Read the model definition and answer for the solid it produces. Units are mm, in the model's axes. A direction names the side the tool comes from. Coordinates: 2 decimals unless noted, no trailing zeros. Write each loop counter-clockwise with the first axis right and the second up, starting at its lowest first coordinate (ties: lowest second). Pieces come first, ordered by that corner, then holes. Notation, with made-up numbers: M 55,31.5 L 81,31.5 A22 ccw 81,41.5 Z; hole C 8,-35 d4. An arc over 180 degrees is marked long. Write item = value, one per line.
from build123d import *

# Parameters (mm, degrees)
F0_R     = 4.5
F1_DEPTH = 8
F2_W     = 22
F2_H     = 60
F2_R     = 2.5
F3_DEPTH = 6
F4_SIZE  = 1


with BuildPart() as f1:
    # F0 (on Right) → F1 (new body, symmetric)
    with BuildSketch(Plane.YZ):
        with BuildLine():
            Line((-30, 10), (-10.925823, -10.27747))
            ThreePointArc((-10.925823, -10.27747), (0, -15), (10.925823, -10.27747))
            Line((10.925823, -10.27747), (30, 10))
            Line((30, 10), (30, 20))
            Line((30, 20), (0, 20))
            Line((0, 20), (-30, 20))
            Line((-30, 20), (-30, 10))
        make_face()
        Circle(F0_R, mode=Mode.SUBTRACT)
    extrude(amount=F1_DEPTH, both=True)

    # F2 (on face) → F3 (join)
    with BuildSketch(Plane.XY.offset(20)):
        Polygon((8, 30), (0, 30), (-8, 30), (-8, -30), (8, -30), align=None)
        with Locations((19, 0)):
            Rectangle(F2_W, F2_H)
        with Locations((20, -20)):
            Circle(F2_R, mode=Mode.SUBTRACT)
        with Locations((20, 20)):
            Circle(F2_R, mode=Mode.SUBTRACT)
        with Locations((-19, 0)):
            Rectangle(F2_W, F2_H)
        with Locations((-20, -20)):
            Circle(F2_R, mode=Mode.SUBTRACT)
        with Locations((-20, 20)):
            Circle(F2_R, mode=Mode.SUBTRACT)
    extrude(amount=F3_DEPTH)

    # F4
    f4_edges = [f1.edges().sort_by_distance(p)[0] for p in [
        (0, 30, 26),
        (-30, 0, 26),
        (0, -30, 26),
        (30, 0, 26),
        (17.5, 20, 26),
        (17.5, -20, 26),
        (-22.5, 20, 26),
        (-22.5, -20, 26),
    ]]
    chamfer(f4_edges, length=F4_SIZE)


solid = f1.part
Item 1: Consider line 1 along Y through (x, z) = (20, 23.95); line 2 along Z through (x, y) = (21.5, -27); line 3 along Z through (x, y) = (-6, -1). Determine where each line is inside the solid, lowest interval first. Write a range as from..to.
Worked answers:
line_1 = -30..-22.5, -17.5..17.5, 22.5..30
line_2 = 20..26
line_3 = -14.97..-4.39, 4.39..26
Item 2: Flat-ended cylindrical pins translate along their axes: pin 1 (2 mm diameter, centred on x = 6.5, y = 20, fed in from -Z); pin 2 (6.5 mm diameter, centred on x = 21, y = -12, fed in from -Z); pin 3 (8 mm diameter, centred on y = 10, z = -9.5, fed in from +X); pin 4 (8 mm diameter, centred on x = -20, y = -20, fed in from +Z). Find the tip coordinate at first contact, or state that the pin passes through.
Worked answers:
pin_1 = -1.69
pin_2 = 20
pin_3 = 8
pin_4 = 26
Item 3: For a pull along X with two mould halves and no side action, classify faces 4 (the face through (-8, 0, 7)), 5 (the face through (-21.84, 21.69, 22.46)), 6 (the face through (0, -30, 19)), 7 (the face through (30, 0, 22)) as released by +X, released by -X, zero draft, split by the parting line, or undercut.
Worked answers:
face_4 = released by -X
face_5 = undercut
face_6 = zero draft
face_7 = released by +X
Item 4: Which of the six approach directions +Z, -Z, +X, -X, +Y, -Y give full straight-line access (tool end or side, diameter ignored) to faces 1 (the face through (-19, 0, 20)), 2 (the face through (8, 0, 7)), 3 (the face through (-30, 0, 22))?
Worked answers:
face_1 = -Z, -X, +Y, -Y
face_2 = -Z, +X, +Y, -Y
face_3 = +Z, -Z, -X, +Y, -Y
Item 5: Find section D-D (z = 1). Determine the outline of the cut face in (x, y), and give its area (3 significant figures).
Worked answers:
outline = M -8,-21.53 L 8,-21.53 L 8,-4.39 L -8,-4.39 Z; M -8,4.39 L 8,4.39 L 8,21.53 L -8,21.53 Z
area = 549 mm²
Item 6: Find section B-B (z = 21). Determine the outline of the cut face in (x, y), and give its area (3 significant figures).
Worked answers:
outline = M -30,-30 L 30,-30 L 30,30 L -30,30 Z; hole C -20,-20 d5; hole C -20,20 d5; hole C 20,-20 d5; hole C 20,20 d5
area = 3,520 mm²
Item 7: Find section C-C (x = 3). Determine the outline of the cut face in (y, z), and give its area (3 significant figures).
Worked answers:
outline = M -30,10 L -10.93,-10.28 A15 ccw 10.93,-10.28 L 30,10 L 30,25 L 29,26 L -29,26 L -30,25 Z; hole C 0,0 d9
area = 1,800 mm²
Item 8: Find section A-A (x = -20). Determine the outline of the cut face in (y, z).
Worked answers:
outline = M -30,20 L -22.5,20 L -22.5,25 L -23.5,26 L -29,26 L -30,25 Z; M -17.5,20 L 17.5,20 L 17.5,25 L 16.5,26 L -16.5,26 L -17.5,25 Z; M 22.5,20 L 30,20 L 30,25 L 29,26 L 23.5,26 L 22.5,25 Z
